Read the model definition and answer for the solid it produces. Units are mm, in the model's axes. Coordinates: 2 decimals unless noted, no trailing zeros. Loops run counter-clockwise (first coordinate to the right, second up) from the corner with the lowest first, then second, coordinate; pieces in that order, holes last. Notation, with made-up numbers: (61.25, 43.5) - (102.25, 43.5) arc R31 ccw to (102.25, 78.5) - close; hole circle Ø11 at (58.5, 32). An arc over 180 degrees is marked (long way). One line per item, written item: value. Start each with the question number.
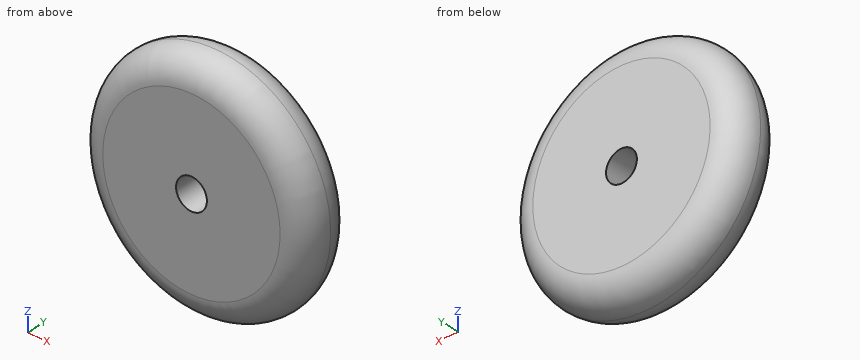
from build123d import *

# Parameters (mm, degrees)
F0_R     = 30
F1_DEPTH = 14
F2_R     = 6.99999
F4_D     = 8
F4_DEPTH = 100
F4_TIP   = 2.4034424761


# Not quite as in the source:
# - a fillet or chamfer is up to 0.001 mm smaller than in the source, because OpenCascade refuses the exact size


with BuildPart() as f1:
    # F0 (on Front) → F1 (new body)
    with BuildSketch(Plane.XZ):
        Circle(F0_R)
    extrude(amount=F1_DEPTH)

    # F2 (radius 7 in the source; OpenCascade refuses exactly that, so slightly less here)
    f2_edges = [f1.edges().sort_by_distance(p)[0] for p in [
        (-30, -14, 0),
        (-30, 0, 0),
    ]]
    fillet(f2_edges, radius=F2_R)

    # F4
    with Locations(Plane(origin=(0, 0, 0), x_dir=(-1, 0, 0), z_dir=(0, 1, 0))):
        with Locations((0, 0)):
            Hole(F4_D / 2, depth=F4_DEPTH)
            with Locations((0, 0, -(F4_DEPTH + F4_TIP / 2))):  # 118° drill point
                Cone(0, F4_D / 2, F4_TIP, mode=Mode.SUBTRACT)


solid = f1.part
1) Flat-ended cylindrical pins translate along their axes: P1, Ø1, axis at y = -8, z = 1.5, coming from the -X side; P2, Ø1, axis at x = -10.5, y = -7, coming from the +Z side; P3, Ø4, axis at y = -1.5, z = 20, coming from the -X side. Find the tip coordinate at first contact, or state that the pin passes through.
2) Straight lines are drawn through the part: L1, parallel to X at y = -8.75, z = 1; L2, parallel to X at y = -12.25, z = 0.5; L3, parallel to Z at x = 0, y = -10.75. For each, find the intervals that lie inside material, in ascending order.
3) Section C-C, the plane y = -7.75 is taken. Determine the outline of the cut face in (x, z).
4) Section D-D, the plane y = -12 is taken. Determine the outline of the cut face in (x, z), and give its area (4 significant figures).
Answer below:
1. P1: x = -29.95
1. P2: z = 28.28
1. P3: x = -21.85
2. L1: -29.76 to -3.87, 3.87 to 29.76
2. L2: -27.63 to -3.97, 3.97 to 27.63
2. L3: -28.91 to -4, 4 to 28.91
3. outline: circle Ø59.92 at (0, 0); hole circle Ø8 at (0, 0)
4. outline: circle Ø55.8 at (0, 0); hole circle Ø8 at (0, 0)
4. area: 2,395 mm2
